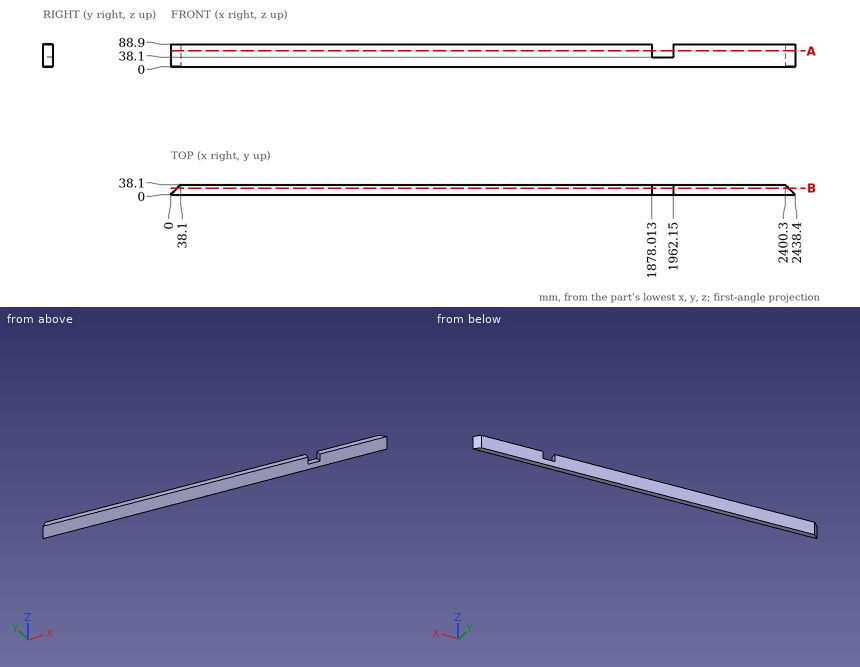
Part print with two shaded views. Sizes in mm from the minimum x, y, z corner. Give positions to 0.01 mm unless a question says otherwise; leave off trailing zeros. Loops run counter-clockwise (first coordinate to the right, second up) from the corner with the lowest first, then second, coordinate; pieces in that order, holes last. Notation, with made-up numbers: (69, -14) -> (93, -14) arc R22 cw to (93, -8) -> close; hole circle Ø11 at (25, -30). An arc over 180 degrees is marked (long way). One line per question, with ' | ' between items.
Q1. Cut at B-B, the plane y = 24.5. Write the cut outline in (x, z), plus the area to 3 significant figures.
Filled sheet:
outline: (24.5, 0) -> (2413.9, 0) -> (2413.9, 88.9) -> (1962.15, 88.9) -> (1962.15, 38.1) -> (1878.01, 38.1) -> (1878.01, 88.9) -> (24.5, 88.9) -> close | area: 208,000 mm²
Q2. Drill centre lines: line 1 along X through (y, z) = (14, 5.5); line 2 along X through (y, z) = (10, 8). Where is each one in solid material? Low to high. Write a range as [from, to].
Filled sheet:
line 1: x = [14, 2424.4] | line 2: x = [10, 2428.4]
Q3. Cut at A-A, the plane z = 62.5. Write the cut outline in (x, y).
Filled sheet:
outline: (0, 0) -> (1878.01, 0) -> (1878.01, 38.1) -> (38.1, 38.1) -> close; (1962.15, 0) -> (2438.4, 0) -> (2400.3, 38.1) -> (1962.15, 38.1) -> close
Q4. Drop flat-ended pins along their axis: pin 1 (10 mm diameter, centred on y = 19.5, z = 44, fed in from +X); pin 2 (3 mm diameter, centred on y = 23, z = 23, fed in from -X); pin 3 (4 mm diameter, centred on y = 21.5, z = 40, fed in from -X). Give the stop position or say it passes through.
Filled sheet:
pin 1: stops at x = 2423.9 | pin 2: stops at x = 21.5 | pin 3: stops at x = 19.5
